Build history of the part. All positions in model axes, mm. A direction names the side the tool comes from. Give positions to 0.01 mm unless a question says otherwise; leave off trailing zeros. Order: outer loops, then holes, each group sorted by start corner. A loop starts at its lowest first (then second) coordinate and runs counter-clockwise, first axis right, second up. Notation, with made-up numbers: (32.25, 81.5) - (83.25, 81.5) arc R21 cw to (83.25, 106.5) - close; hole circle Ø1 at (-16.75, -13.75). An arc over 180 degrees is marked (long way). One line per item, written item: value.
```python
from build123d import *

# Parameters (mm, degrees)
F0_W      = 56.428283453
F0_H      = 121.9848245382
F1_DEPTH  = 6.35
F2_W      = 13.6921107769
F2_H      = 87.1320217848
F3_DEPTH  = 12.7
F4_W      = 12.7
F4_H      = 12.6656033099
F5_DEPTH  = 152.4
F6_W      = 12.7
F6_H      = 13.4637728333
F7_DEPTH  = 152.4
F8_R      = 3.224201557
F8_R_2    = 2.7149600872
F9_DEPTH  = 6.351
F10_W     = 247.7097766638
F10_H     = 86.6629034281
F11_DEPTH = 6.35
F12_W     = 14.8840993643
F12_H     = 44.3546175957
F12_W_2   = 15.5743807554
F12_H_2   = 78.4596502781
F13_DEPTH = 25.4
F14_R     = 5.08
F15_DEPTH = 5.08


# Not quite as in the source:
# - the program builds the solid bodies; features that only make, move or delete a surface that nothing else refers to are left out


with BuildPart() as f1:
    # F0 (on Front) → F1 (new body)
    with BuildSketch(Plane.XZ):
        Rectangle(F0_W, F0_H)
    extrude(amount=F1_DEPTH)

    # F2 (on face) → F3 (join)
    with BuildSketch(Plane.XZ.offset(6.35)):
        Rectangle(F2_W, F2_H)
    extrude(amount=F3_DEPTH)

    # F4 (on face) → F5 (join)
    with BuildSketch(Plane.YZ.offset(6.8460553885)):
        with Locations((-12.7, 37.2332092375)):
            Rectangle(F4_W, F4_H)
    extrude(amount=F5_DEPTH)

    # F6 (on face) → F7 (join)
    with BuildSketch(Plane.YZ.offset(6.8460553885)):
        with Locations((-12.7, -36.8341244757)):
            Rectangle(F6_W, F6_H)
    extrude(amount=F7_DEPTH)

    # F8 (on face) → F9 (cut, through all)
    with BuildSketch(Plane.XZ.offset(6.35)):
        with Locations((0, 52.0230680704)):
            Circle(F8_R)
        with Locations((0, -52.8460629284)):
            Circle(F8_R_2)
    extrude(amount=-F9_DEPTH, mode=Mode.SUBTRACT)

    # F10 (on face) → F11 (join)
    with BuildSketch(Plane.YZ.offset(159.2460553885)):
        with Locations((-130.2048883319, 0.2345591784)):
            Rectangle(F10_W, F10_H)
    extrude(amount=F11_DEPTH)

    # F12 (on face) → F13 (cut)
    with BuildSketch(Plane.YZ.offset(165.5960553885)):
        with Locations((-55.5786713958, 33.0530032516)):
            Rectangle(F12_W, F12_H)
        with Locations((-205.3182795644, 27.350962162)):
            Rectangle(F12_W_2, F12_H_2)
    extrude(amount=-F13_DEPTH, mode=Mode.SUBTRACT)

    # F14
    f14_edges = [f1.edges().sort_by_distance(p)[0] for p in [
        (162.421055, -254.059777, 43.566011),
        (162.421055, -254.059777, -43.096893),
    ]]
    fillet(f14_edges, radius=F14_R)

    # F15 (add): a face of the model
    f15_faces = [f1.faces().sort_by_distance(p)[0] for p in [
        (0, 0, -0.0696069338),
    ]]
    extrude(f15_faces, amount=F15_DEPTH)


solid = f1.part
```
(1) Slice it at A-A, the plane x = 113. Give the cut face in (y, z).
Completed:
outline: (-19.05, -43.57) - (-6.35, -43.57) - (-6.35, -30.1) - (-19.05, -30.1) - close; (-19.05, 30.9) - (-6.35, 30.9) - (-6.35, 43.57) - (-19.05, 43.57) - close
(2) Pin check, flat tips, straight feed: P1, Ø5, axis at x = 162.5, y = -179.5, coming from the -Z side; P2, Ø2, axis at x = 82, z = -27.5, coming from the +Y side; P3, Ø6.5, axis at x = 35.5, y = -9.5, coming from the -Z side; P4, Ø3, axis at x = 163.5, y = -123, coming from the +Z side. Stop position of each tip, or through.
Completed:
P1: z = -43.1
P2: through
P3: z = -43.57
P4: z = 43.57
(3) Slice it at C-C, the plane z = -26.5. Give the cut face in (x, y).
Completed:
outline: (-28.21, -6.35) - (-6.85, -6.35) - (-6.85, -19.05) - (6.85, -19.05) - (6.85, -6.35) - (28.21, -6.35) - (28.21, 5.08) - (-28.21, 5.08) - close; (159.25, -254.06) - (165.6, -254.06) - (165.6, -6.35) - (159.25, -6.35) - close
(4) Drill centre lines: line 1 (Z direction, x = 0, y = 0); line 2 (Y direction, x = 16, z = -36); line 3 (Z direction, x = 39.5, y = -9). Where is each one in solid material? Low to high.
Completed:
line 1: -60.99 to -55.56, -50.13 to 48.8, 55.25 to 60.99
line 2: -19.05 to 5.08
line 3: -43.57 to -30.1, 30.9 to 43.57
(5) Slice it at D-D, the plane y = -202. Give the cut face in (x, z).
Completed:
outline: (159.25, -43.1) - (165.6, -43.1) - (165.6, -11.88) - (159.25, -11.88) - close
(6) Pull direction X, two halves, no side cores. Call faces 4 (the face through (102, -6.35, 32)), 5 (the face through (1.253, -0.715, -55.255)), 6 (the face through (-6.846, -13, -1)): +X half, -X half, draft (parallel to the pull), parting line (faces both ways), or undercut.
Completed:
face 4: draft
face 5: undercut
face 6: -X half
(7) 3-axis set-ups, long thin cutter, end or side, ignore diameter. For faces 1 (the face through (28.214, -1, -1)), 2 (the face through (6.846, -13, 0)), 3 (the face through (162, -197.531, 15)): which of +Z, -Z, +X, -X, +Y, -Y reach the whole face in a straight line?
Completed:
face 1: +Z, -Z, +X, +Y
face 2: -Y
face 3: +Z, +X, -X
(8) Slice it at B-B, the plane z = 16. Give the cut face in (x, y).
Completed:
outline: (-28.21, -6.35) - (-6.85, -6.35) - (-6.85, -19.05) - (6.85, -19.05) - (6.85, -6.35) - (28.21, -6.35) - (28.21, 5.08) - (-28.21, 5.08) - close; (159.25, -254.06) - (165.6, -254.06) - (165.6, -213.11) - (159.25, -213.11) - close; (159.25, -197.53) - (165.6, -197.53) - (165.6, -63.02) - (159.25, -63.02) - close; (159.25, -48.14) - (165.6, -48.14) - (165.6, -6.35) - (159.25, -6.35) - close
